from build123d import *

# Parameters (mm, degrees)
SKETCH_1_W          = 15
SKETCH_1_H          = 15
SKETCH_1_W_2        = 13
SKETCH_1_H_2        = 13
EXTRUDE_1_DEPTH     = 520
SKETCH_2_R          = 1.6
CUT_EXTRUDE_1_DEPTH = 521.270362408
SKETCH_3_R          = 1.6
CUT_EXTRUDE_2_DEPTH = 521.270362408


with BuildPart() as part:
    # 草图1 → 拉伸-薄壁1 (new body)
    with BuildSketch(Plane(origin=(0, 0, 0), x_dir=(1, 0, 0), z_dir=(0, 1, 0))):
        Rectangle(SKETCH_1_W, SKETCH_1_H)
        Rectangle(SKETCH_1_W_2, SKETCH_1_H_2, mode=Mode.SUBTRACT)
    extrude(amount=EXTRUDE_1_DEPTH)

    # 草图2 → 切除-拉伸1 (cut, through all)
    with BuildSketch(Plane.XY.offset(7.5)):
        with Locations((0, 7.5)):
            Circle(SKETCH_2_R)
        with Locations((0, 27.5)):
            Circle(SKETCH_2_R)
        with Locations((0, 75)):
            Circle(SKETCH_2_R)
        with Locations((0, 95)):
            Circle(SKETCH_2_R)
        with Locations((0, 115)):
            Circle(SKETCH_2_R)
        with Locations(Location((0, 405, 0), (0, 0, 180))):
            Circle(SKETCH_2_R)
        with Locations(Location((0, 425, 0), (0, 0, 180))):
            Circle(SKETCH_2_R)
        with Locations(Location((0, 445, 0), (0, 0, 180))):
            Circle(SKETCH_2_R)
        with Locations(Location((0, 492.5, 0), (0, 0, 180))):
            Circle(SKETCH_2_R)
        with Locations(Location((0, 512.5, 0), (0, 0, 180))):
            Circle(SKETCH_2_R)
    extrude(amount=-CUT_EXTRUDE_1_DEPTH, mode=Mode.SUBTRACT)

    # 草图3 → 切除-拉伸2 (cut, through all)
    with BuildSketch(Plane(origin=(7.5, 0, 0), x_dir=(0, 0, -1), z_dir=(1, 0, 0))):
        with Locations((0, 20)):
            Circle(SKETCH_3_R)
        with Locations((0, 70)):
            Circle(SKETCH_3_R)
        with Locations((0, 450)):
            Circle(SKETCH_3_R)
        with Locations((0, 500)):
            Circle(SKETCH_3_R)
    extrude(amount=-CUT_EXTRUDE_2_DEPTH, mode=Mode.SUBTRACT)


solid = part.part
CAD build for the part. Positions are in the model's coordinates, mm. A direction names the side the tool comes from. Round coordinates to 2 decimals unless told otherwise and drop trailing zeros. Write each loop counter-clockwise with the first axis right and the second up, starting at its lowest first coordinate (ties: lowest second). Pieces come first, ordered by that corner, then holes. Notation, with made-up numbers: M 69.5,-8.5 L 87.5,-8.5 A31 cw 87.5,22.5 Z; hole C 1,31.25 d1. An arc over 180 degrees is marked long. Put each result on its own line as item: value. Start each with the question number.
1) 3-axis set-ups, long thin cutter, end or side, ignore diameter. For faces 1 (the flat face through (-6.5, 256, 0)), 2 (the flat face through (0, 256, -7.5)): which of +Z, -Z, +X, -X, +Y, -Y reach the whole face in a straight line?
2) Pull direction X, two halves, no side cores. Call faces 3 (the flat face through (6.5, 256, 0)), 4 (the flat face through (0, 256, 7.5)), 5 (the flat face through (0, 256, 6.5)), 6 (the flat face through (-7.5, 256, 0)): pulls with the +X half, pulls with the -X half, needs draft (parallel to the pull), parting line crosses it, or undercut.
3) Saw through at A-A, the plane y = 314.5. Write the cut outline in (x, z).
4) Drill centre lines: probe 1 along Y at (x, z) = (6.7, 0); probe 2 along Z at (x, y) = (-1.25, 476). Where is each one in solid material? Low to high. Write a range as [from, to].
Resolved:
1. face 1: +Y, -Y
1. face 2: -Z, +X, -X, +Y, -Y
2. face 3: undercut
2. face 4: needs draft
2. face 5: undercut
2. face 6: pulls with the -X half
3. outline: M -7.5,-7.5 L 7.5,-7.5 L 7.5,7.5 L -7.5,7.5 Z; hole M -6.5,-6.5 L 6.5,-6.5 L 6.5,6.5 L -6.5,6.5 Z
4. probe 1: [0, 18.4], [21.6, 68.4], [71.6, 448.4], [451.6, 498.4], [501.6, 520]
4. probe 2: [-7.5, -6.5], [6.5, 7.5]
